Design review of the part built by this model. Coordinates are the model's own, in mm. A direction names the side the tool comes from. Coordinates: 2 decimals unless noted, no trailing zeros. Loops run counter-clockwise (first coordinate to the right, second up) from the corner with the lowest first, then second, coordinate; pieces in that order, holes last. Notation, with made-up numbers: (48, 7) -> (65, 7) arc R7 cw to (65, 12) -> close; hole circle Ø5 at (-1, 7.25). An arc over 180 degrees is marked (long way). Answer as a JSON object with one key per item and string values.
```python
from build123d import *

# Parameters (mm, degrees)
F2_DEPTH  = 3
F0_R      = 11.75
F3_DEPTH  = 7.9
F4_DEPTH  = 7.9
F5_DEPTH  = 3
F6_R      = 5
F6_2_R    = 5
F9_D      = 3
F10_DEPTH = 4
F11_DEPTH = 4


with BuildPart() as f2:
    # F0 (on Top) → F2 (new body)
    with BuildSketch(Plane.XY):
        with BuildLine():
            ThreePointArc((70.8448413014, 3.4252903424), (76.5230858808, 21.4851908555), (86, 37.8739237785))
            Line((86, 37.8739237785), (-65.6162592679, 37.8739237785))
            ThreePointArc((-65.6162592679, 37.8739237785), (-82.3199649398, 11.4193737584), (-82.519158721, -19.8666825891))
            Line((-82.519158721, -19.8666825891), (-73.9695476283, -37.2867286205))
            Line((-73.9695476283, -37.2867286205), (86, -37.2867286205))
            ThreePointArc((86, -37.2867286205), (77.4631412951, -21.4263167299), (71.2877699379, -4.5060504646))
            ThreePointArc((71.2877699379, -4.5060504646), (70.5487291916, -0.5692843065), (70.8448413014, 3.4252903424))
        make_face()
    extrude(amount=-F2_DEPTH)


with BuildPart() as f3:
    # F0 (on Top) → F3 (new body)
    with BuildSketch(Plane.XY):
        with BuildLine():
            ThreePointArc((-82.519158721, -19.8666825891), (-82.3199649398, 11.4193737584), (-65.6162592679, 37.8739237785))
            Line((-65.6162592679, 37.8739237785), (-99.2088739193, 37.8739237785))
            ThreePointArc((-99.2088739193, 37.8739237785), (-117.1879721114, 26.6373104948), (-114.9666717313, 5.5523567478))
            Line((-114.9666717313, 5.5523567478), (-81.4747432756, -37.2867286205))
            Line((-81.4747432756, -37.2867286205), (-73.9695476283, -37.2867286205))
            Line((-73.9695476283, -37.2867286205), (-82.519158721, -19.8666825891))
        make_face()
        with Locations((-99.2088739193, 17.8719250206)):
            Circle(F0_R, mode=Mode.SUBTRACT)
    extrude(amount=F3_DEPTH)


with BuildPart() as f4:
    # F0 (on Top) → F4 (new body)
    with BuildSketch(Plane.XY):
        with BuildLine():
            Line((86, -37.2867286205), (86, 37.8739237785))
            ThreePointArc((86, 37.8739237785), (76.5230858808, 21.4851908555), (70.8448413014, 3.4252903424))
            ThreePointArc((70.8448413014, 3.4252903424), (70.5487291916, -0.5692843065), (71.2877699379, -4.5060504646))
            ThreePointArc((71.2877699379, -4.5060504646), (77.4631412951, -21.4263167299), (86, -37.2867286205))
        make_face()
    extrude(amount=F4_DEPTH)


with BuildPart() as f5:
    # F5 (new): a face of the model
    f5_faces = [f3.part.faces().sort_by_distance(p)[0] for p in [
        (-83.2059045041, 11.6787223922, 0),
    ]]
    extrude(f5_faces, amount=F5_DEPTH)

    # F6#2
    f6_2_edges = [f5.edges().sort_by_distance(p)[0] for p in [
        (-81.474743, -37.286729, -1.5),
    ]]
    fillet(f6_2_edges, radius=F6_2_R)


with BuildPart() as f5b:
    # F5#2 (new): a face of the model
    f5_2_faces = [f4.part.faces().sort_by_distance(p)[0] for p in [
        (80.189714527, 0.7740894227, 0),
    ]]
    extrude(f5_2_faces, amount=F5_DEPTH)


with BuildPart() as f3_1:
    add(f3.part)

    # F6
    f6_edges = [f3_1.edges().sort_by_distance(p)[0] for p in [
        (-81.474743, -37.286729, 3.95),
    ]]
    fillet(f6_edges, radius=F6_R)


with BuildPart() as f2_1:
    add(f2.part)

    # F7: union F3, F4, F5, F5b
    add(f3_1.part)
    add(f4.part)
    add(f5.part)
    add(f5b.part)

    # F9 (through all)
    with Locations(Plane(origin=(0, 0, -3), x_dir=(1, 0, 0), z_dir=(0, 0, -1))):
        with Locations((-81.1894536018, 31.5095931292), (-113.9387488365, -24.5540793985), (-76.3550326228, -33.2092493773), (82.3921039701, 23.663148284), (82.3921039701, -25.700064376)):
            Hole(F9_D / 2)

    # F8 (on face) → F10 (cut)
    with BuildSketch(Plane(origin=(0, 0, -3), x_dir=(1, 0, 0), z_dir=(0, 0, -1))):
        Polygon((-74.5737203647, -36.1802637897), (-72.8914025376, -33.1520949158), (-74.6727147957, -30.1810805034), (-78.136344881, -30.2382349648), (-79.8186627081, -33.2664038387), (-78.0373504499, -36.2374182511), align=None)
        Polygon((85.3921039701, 21.9310974764), (85.3921039701, 25.3951990915), (82.3921039701, 27.1272498991), (79.3921039701, 25.3951990915), (79.3921039701, 21.9310974764), (82.3921039701, 20.1990466688), align=None)
        Polygon((85.3921039701, -27.4321151836), (85.3921039701, -23.9680135684), (82.3921039701, -22.2359627609), (79.3921039701, -23.9680135684), (79.3921039701, -27.4321151836), (82.3921039701, -29.1641659911), align=None)
        Polygon((-79.8767595984, 28.3038429122), (-77.7568454741, 31.043544375), (-79.0695394775, 34.249294592), (-82.5021476052, 34.7153433461), (-84.6220617296, 31.9756418833), (-83.3093677262, 28.7698916664), align=None)
        Polygon((-110.4805015339, -24.7553890954), (-112.0352858737, -21.6598042304), (-115.4935331763, -21.4584945334), (-117.3969961391, -24.3527697016), (-115.8422117994, -27.4483545667), (-112.3839644968, -27.6496642636), align=None)
    extrude(amount=-F10_DEPTH, mode=Mode.SUBTRACT)

    # F8 (on face) → F11 (cut)
    with BuildSketch(Plane(origin=(0, 0, -3), x_dir=(1, 0, 0), z_dir=(0, 0, -1))):
        Polygon((-74.5737203647, -36.1802637897), (-72.8914025376, -33.1520949158), (-74.6727147957, -30.1810805034), (-78.136344881, -30.2382349648), (-79.8186627081, -33.2664038387), (-78.0373504499, -36.2374182511), align=None)
        Polygon((85.3921039701, 21.9310974764), (85.3921039701, 25.3951990915), (82.3921039701, 27.1272498991), (79.3921039701, 25.3951990915), (79.3921039701, 21.9310974764), (82.3921039701, 20.1990466688), align=None)
        Polygon((85.3921039701, -27.4321151836), (85.3921039701, -23.9680135684), (82.3921039701, -22.2359627609), (79.3921039701, -23.9680135684), (79.3921039701, -27.4321151836), (82.3921039701, -29.1641659911), align=None)
        Polygon((-79.8767595984, 28.3038429122), (-77.7568454741, 31.043544375), (-79.0695394775, 34.249294592), (-82.5021476052, 34.7153433461), (-84.6220617296, 31.9756418833), (-83.3093677262, 28.7698916664), align=None)
        Polygon((-110.4805015339, -24.7553890954), (-112.0352858737, -21.6598042304), (-115.4935331763, -21.4584945334), (-117.3969961391, -24.3527697016), (-115.8422117994, -27.4483545667), (-112.3839644968, -27.6496642636), align=None)
    extrude(amount=-F11_DEPTH, mode=Mode.SUBTRACT)


solid = f2_1.part
```
1) For faces 4 (the flat face through (-46, 37.874, -1)), 5 (the flat face through (-78.185, -28.699, 3.895)), 6 (the flat face through (-87, 9, 7.9)), 7 (the cylindrical face through (77.36, -21.2, 3.89)), 8 (the flat face through (-75, 32, 1)), list the 3-axis set-ups (+Z, -Z, +X, -X, +Y, -Y) from which the entire face can be reached by the end or side of a thin tool; tool diameter is ignored.
Completed:
{"face 4": "+Z, -Z, +X, -X, +Y", "face 5": "+Z", "face 6": "+Z, +X, -X, +Y, -Y", "face 7": "+Z, -Y", "face 8": "-Z"}
2) Add section B-B, the plane y = -18. Give the boundary of the cut face in (x, z).
Completed:
{"outline": "(-96.55, -3) -> (86, -3) -> (86, 7.9) -> (75.99, 7.9) -> (75.99, 0) -> (-83.01, 0) -> (-83.01, 7.9) -> (-96.55, 7.9) -> close"}
3) Add section A-A, the plane z = 5. Give the boundary of the cut face in (x, y), and give its area (3 significant figures).
Completed:
{"outline": "(-114.97, 5.55) -> (-82.98, -35.37) arc R5 ccw to (-79.04, -37.29) -> (-73.97, -37.29) -> (-82.52, -19.87) arc R56.92 cw to (-65.62, 37.87) -> (-99.21, 37.87) arc R20 ccw to start; (70.84, 3.43) arc R15.48 ccw to (71.29, -4.51) arc R125.34 ccw to (86, -37.29) -> (86, 37.87) arc R86.36 ccw to start; hole circle Ø3 at (-113.94, 24.55); hole circle Ø23.5 at (-99.21, 17.87); hole circle Ø3 at (-81.19, -31.51); hole circle Ø3 at (-76.36, 33.21); hole circle Ø3 at (82.39, -23.66); hole circle Ø3 at (82.39, 25.7)", "area": "2,200 mm²"}
4) Add section C-C, the plane x = -68. Give the boundary of the cut face in (y, z).
Completed:
{"outline": "(-37.29, -3) -> (37.87, -3) -> (37.87, 7.9) -> (35.62, 7.9) -> (35.62, 0) -> (-37.29, 0) -> close"}
5) Wall thickness on probe 1 along X at (y, z) = (-24.5, 7.5); probe 2 along Y at (x, z) = (-77.5, 5); probe 3 along X at (y, z) = (33, 0.5): over which ranges is each line inside the solid? List them lowest first.
Completed:
{"probe 1": "-91.47 to -80.25, 78.89 to 81.15, 83.64 to 86", "probe 2": "-37.29 to -30.09, 22.98 to 32.24, 34.18 to 37.87", "probe 3": "-112.29 to -79.67, -72.98 to -70.45, 82.67 to 86"}
6) The part is to be moulded in two halves that separate along X. For faces 1 (the flat face through (-18, 1, -3)), 2 (the flat face through (-1, 1, 0)), 3 (the cylindrical face through (-81.2, -36.795, 2.374)), say which applies: pulls with the +X half, pulls with the -X half, needs draft (parallel to the pull), parting line crosses it, or undercut.
Completed:
{"face 1": "needs draft", "face 2": "undercut", "face 3": "pulls with the -X half"}
7) Clearance check with flat-ended pins moving along their axes: pin 1 Ø3 at (x, y) = (82, 24) entering from -Z; pin 2 Ø3 at (y, z) = (-24.5, -1) entering from -X; pin 3 Ø22.5 at (x, y) = (21.5, 5.5) entering from +Z; pin 4 Ø5 at (x, y) = (-114, 24.5) entering from -Z. State where each tip first meets the part, or that it passes through.
Completed:
{"pin 1": "z = -3", "pin 2": "x = -92.64", "pin 3": "z = 0", "pin 4": "z = 1"}
